from build123d import *

# Parameters (mm, degrees)
F0_W     = 150
F0_H     = 150
F1_DEPTH = 12.7
F2_R     = 4.5
F2_R_2   = 3.75
F3_DEPTH = 12.701


with BuildPart() as f1:
    # F0 (on Front) → F1 (new body)
    with BuildSketch(Plane.XZ):
        Rectangle(F0_W, F0_H)
    extrude(amount=F1_DEPTH)

    # F2 (on Front) → F3 (cut, through all)
    with BuildSketch(Plane.XZ):
        with Locations((-60, 60)):
            Circle(F2_R)
        with Locations((60, 60)):
            Circle(F2_R)
        with Locations((-60, -60)):
            Circle(F2_R)
        with Locations((60, -60)):
            Circle(F2_R)
        with Locations((0, 66)):
            Circle(F2_R_2)
        with Locations((-46.669048, 46.669048)):
            Circle(F2_R_2)
        with Locations((-66, 0)):
            Circle(F2_R_2)
        with Locations((-46.669048, -46.669048)):
            Circle(F2_R_2)
        with Locations((0, -66)):
            Circle(F2_R_2)
        with Locations((46.669048, -46.669048)):
            Circle(F2_R_2)
        with Locations((66, 0)):
            Circle(F2_R_2)
        with Locations((46.669048, 46.669048)):
            Circle(F2_R_2)
    extrude(amount=F3_DEPTH, mode=Mode.SUBTRACT)


solid = f1.part
Could you check a few things on this model? Use its own coordinates, in mm. Give positions to 0.01 mm unless a question says otherwise; leave off trailing zeros. Order: outer loops, then holes, each group sorted by start corner. A loop starts at its lowest first (then second) coordinate and runs counter-clockwise, first axis right, second up.
Item 1: I need wall thicknesses on line 1 (X direction, y = -7.25, z = -60); line 2 (Z direction, x = 0, y = -3). Which ranges of each line are inside material? Lowest first, please.
Item 2: If we section it at C-C, the plane y = -9.5: Count the separate pieces of the cut face and the enclosed holes in it, plus the area to 3 significant figures.
Item 3: I'm going to push a flat-ended pin straight in: pin 1 (7 mm diameter, centred on x = 66, z = 0, fed in from -Y). Where does the tip first touch, or does it pass through?
Item 4: If we section it at A-A, the plane x = -60: Write out the boundary of the cut face in (y, z).
Item 5: If we section it at B-B, the plane z = 0: Write out the boundary of the cut face in (x, y).
Item 6: If we mould it in two halves opening along Z, with no side actions, what happens to faces 1 (the face through (-75, -6, -1)), 2 (the face through (-0.488, -6.261, -62.282)), 3 (the face through (-1, -6, -75))? For each: pulls with the +Z half, pulls with the -Z half, needs draft (parallel to the pull), parting line crosses it, or undercut.
Values:
1. line 1: x = -75 to -64.5, -55.5 to 55.5, 64.5 to 75
1. line 2: z = -75 to -69.75, -62.25 to 62.25, 69.75 to 75
2. separate pieces: 1
2. enclosed holes: 12
2. area: 21,900 mm2
3. pin 1: passes through
4. outline: (-12.7, -75) - (0, -75) - (0, -64.5) - (-12.7, -64.5) - close; (-12.7, -55.5) - (0, -55.5) - (0, 55.5) - (-12.7, 55.5) - close; (-12.7, 64.5) - (0, 64.5) - (0, 75) - (-12.7, 75) - close
5. outline: (-75, -12.7) - (-69.75, -12.7) - (-69.75, 0) - (-75, 0) - close; (-62.25, -12.7) - (62.25, -12.7) - (62.25, 0) - (-62.25, 0) - close; (69.75, -12.7) - (75, -12.7) - (75, 0) - (69.75, 0) - close
6. face 1: needs draft
6. face 2: undercut
6. face 3: pulls with the -Z half
